from build123d import *

# Parameters (mm, degrees)
F0_W     = 216.278978
F0_H     = 298.947731
F1_DEPTH = 25.4
F3_DEPTH = 25.401
F4_R     = 5.08


with BuildPart() as f1:
    # F0 (on Front) → F1 (new body)
    with BuildSketch(Plane.XZ):
        with Locations((219.096657, -169.175098)):
            Rectangle(F0_W, F0_H)
        with BuildLine():
            Line((184.616528, -238.748165), (130.02329, -238.748165))
            ThreePointArc((130.02329, -238.748165), (126.474409, -237.364118), (124.799581, -233.942848))
            Line((124.799581, -233.942848), (118.633306, -160.167299))
            ThreePointArc((118.633306, -160.167299), (118.61527, -159.687422), (118.641226, -159.207907))
            Line((118.641226, -159.207907), (123.846745, -107.272929))
            ThreePointArc((123.846745, -107.272929), (124.240313, -105.74049), (125.073194, -104.395284))
            Line((125.073194, -104.395284), (133.473927, -94.539658))
            ThreePointArc((133.473927, -94.539658), (135.266342, -93.180753), (137.463267, -92.698165))
            Line((137.463267, -92.698165), (168.056644, -92.698165))
            ThreePointArc((168.056644, -92.698165), (169.565835, -93.032536), (170.792564, -93.973066))
            Line((170.792564, -93.973066), (180.904666, -106.011276))
            ThreePointArc((180.904666, -106.011276), (181.54046, -106.648087), (182.275801, -107.166771))
            Line((182.275801, -107.166771), (194.915857, -114.54529))
            ThreePointArc((194.915857, -114.54529), (196.686537, -116.243842), (197.490259, -118.562121))
            Line((197.490259, -118.562121), (198.506103, -128.94903))
            ThreePointArc((198.506103, -128.94903), (200.394922, -132.488586), (204.233364, -133.655834))
            Line((204.233364, -133.655834), (214.386911, -132.662812))
            ThreePointArc((214.386911, -132.662812), (218.225352, -133.83006), (220.114172, -137.369617))
            Line((220.114172, -137.369617), (221.566417, -152.21868))
            ThreePointArc((221.566417, -152.21868), (223.26186, -155.591256), (226.783449, -156.950375))
            Line((226.783449, -156.950375), (243.912482, -156.950375))
            ThreePointArc((243.912482, -156.950375), (244.805431, -157.026991), (245.672278, -157.254599))
            Line((245.672278, -157.254599), (263.762319, -163.70189))
            Line((263.762319, -163.70189), (269.194545, -165.637936))
            ThreePointArc((269.194545, -165.637936), (273.975354, -164.984071), (276.196264, -160.700236))
            Line((276.196264, -160.700236), (276.196264, -133.352479))
            ThreePointArc((276.196264, -133.352479), (276.595282, -131.346481), (277.73159, -129.645878))
            Line((277.73159, -129.645878), (286.865628, -120.511846))
            ThreePointArc((286.865628, -120.511846), (288.566229, -119.375541), (290.572226, -118.976524))
            Line((290.572226, -118.976524), (299.14298, -118.976524))
            ThreePointArc((299.14298, -118.976524), (301.0156, -119.322423), (302.641084, -120.314471))
            Line((302.641084, -120.314471), (315.445448, -131.787646))
            ThreePointArc((315.445448, -131.787646), (316.689157, -133.457128), (317.184955, -135.479049))
            Line((317.184955, -135.479049), (320.937758, -227.944813))
            ThreePointArc((320.937758, -227.944813), (319.481155, -231.788052), (315.700147, -233.399309))
            Line((315.700147, -233.399309), (303.73928, -233.399309))
            ThreePointArc((303.73928, -233.399309), (303.098145, -233.359953), (302.466639, -233.242477))
            Line((302.466639, -233.242477), (270.995202, -225.366149))
            ThreePointArc((270.995202, -225.366149), (270.726, -225.306254), (270.45402, -225.260601))
            Line((270.45402, -225.260601), (263.762319, -224.317615))
            Line((263.762319, -224.317615), (223.293336, -218.614775))
            Line((223.293336, -218.614775), (204.573976, -215.976866))
            ThreePointArc((204.573976, -215.976866), (201.545132, -216.45584), (199.302489, -218.547219))
            Line((199.302489, -218.547219), (189.156557, -236.126528))
            ThreePointArc((189.156557, -236.126528), (187.237828, -238.045686), (184.616528, -238.748165))
        make_face(mode=Mode.SUBTRACT)
    extrude(amount=F1_DEPTH)

    # F2 (on face) → F3 (cut, through all)
    with BuildSketch(Plane.XZ.offset(25.4)):
        with BuildLine():
            Line((194.915857, -114.54529), (184.616528, -238.748165))
            Line((184.616528, -238.748165), (235.530938, -238.748165))
            ThreePointArc((235.530938, -238.748165), (240.021066, -236.888293), (241.880938, -232.398165))
            Line((241.880938, -232.398165), (241.880938, -228.548973))
            ThreePointArc((241.880938, -228.548973), (244.068216, -223.753742), (249.123218, -222.261975))
            Line((249.123218, -222.261975), (270.995202, -225.366149))
            Line((270.995202, -225.366149), (270.995202, -172.679961))
            Line((270.995202, -172.679961), (284.431964, -163.976327))
            Line((284.431964, -163.976327), (282.256097, -145.11849))
            Line((282.256097, -145.11849), (194.915857, -114.54529))
        make_face()
    extrude(amount=-F3_DEPTH, mode=Mode.SUBTRACT)

    # F4
    f4_edges = [f1.edges().sort_by_distance(p)[0] for p in [
        (276.196264, -12.7, -142.997263),
    ]]
    fillet(f4_edges, radius=F4_R)


solid = f1.part
Source: CAD feature listing. Evaluate the final solid. Frame: model axes, mm. A direction names the side the tool comes from. Give positions to 0.01 mm unless a question says otherwise; leave off trailing zeros. Write each loop counter-clockwise with the first axis right and the second up, starting at its lowest first coordinate (ties: lowest second). Pieces come first, ordered by that corner, then holes. Notation, with made-up numbers: (31, 41) - (38, 41) arc R14 ccw to (38, 54) - close; hole circle Ø10 at (-35.5, -38). An arc over 180 degrees is marked (long way). Write item = value, one per line. Start each with the question number.
Q1. Material intervals for probe 1 along Z at (x, y) = (271, -21.75); probe 2 along Z at (x, y) = (151.5, -1.25); probe 3 along X at (y, z) = (-10.5, -202), sorted ascending.
Q2. Cut plane B-B, the plane z = -169.5. Return loops of the section in (x, y).
Q3. Draft query along Z for faces 1 (the flat face through (218, -13, -19.701)), 2 (the cylindrical face through (274.11, -12.52, -139.94)), 3 (the flat face through (110.957, -13, -171)). Return one class per face: +Z half, -Z half, draft (parallel to the pull), parting line (faces both ways), or undercut.
Q4. Reachability of faces 4 (the flat face through (182, -13, -238.748)), 5 (the flat face through (266, 0, -134)) from +Z, -Z, +X, -X, +Y, -Y: full face, straight path, thin tool, end or side. Return the list, or none.
Q5. Cut plane A-A, the plane x = 210. Return loops of the section in (y, z), then the cut area to 3 significant figures.
Computed values:
q1.probe_1 = -318.65 to -225.37, -140.92 to -19.7
q1.probe_2 = -318.65 to -238.75, -92.7 to -19.7
q1.probe_3 = 110.96 to 122.13, 319.88 to 327.24
q2.outline = (110.96, -25.4) - (119.41, -25.4) - (119.41, 0) - (110.96, 0) - close; (318.57, -25.4) - (327.24, -25.4) - (327.24, 0) - (318.57, 0) - close
q3.face_1 = +Z half
q3.face_2 = undercut
q3.face_3 = draft
q4.face_4 = +Y, -Y
q4.face_5 = +Z, -Z, +X, -X, +Y
q5.outline = (-25.4, -318.65) - (0, -318.65) - (0, -238.75) - (-25.4, -238.75) - close; (-25.4, -119.83) - (0, -119.83) - (0, -19.7) - (-25.4, -19.7) - close
q5.area = 4,570 mm²
